from build123d import *

# Parameters (mm, degrees)
BOSS_EXTRU_1_DEPTH      = 13
BOSS_EXTRU_2_DEPTH      = 8
ESQUISSE4_R             = 5.5
BOSS_EXTRU_3_DEPTH      = 55
ENL_V_START             = -30
ESQUISSE5_R             = 5.5
ESQUISSE5_R_2           = 3
ENL_V_MAT_EXTRU_1_DEPTH = 30


with BuildPart() as part:
    # Esquisse1 → Boss.-Extru.1 (new body)
    with BuildSketch(Plane.XY):
        with BuildLine():
            Line((10.329521935, 9.6), (71.2270063, 5.135702408))
            ThreePointArc((71.2270063, 5.135702408), (76, 0), (71.2270063, -5.135702408))
            Line((71.2270063, -5.135702408), (10.329521935, -9.6))
            ThreePointArc((10.329521935, -9.6), (0, 0), (10.329521935, 9.6))
        make_face()
    extrude(amount=BOSS_EXTRU_1_DEPTH)

    # Esquisse3 → Boss.-Extru.2 (add)
    with BuildSketch(Plane.XY.offset(13)):
        with BuildLine():
            Line((71.263562407, 5.634364269), (10.366078041, 10.09866186))
            ThreePointArc((10.366078041, 10.09866186), (-0.5, 0), (10.366078041, -10.09866186))
            Line((10.366078041, -10.09866186), (71.263562407, -5.634364269))
            ThreePointArc((71.263562407, -5.634364269), (76.5, 0), (71.263562407, 5.634364269))
        make_face()
    extrude(amount=BOSS_EXTRU_2_DEPTH)

    # Esquisse4 → Boss.-Extru.3 (add)
    with BuildSketch(Plane.XY.offset(21)):
        with Locations((9.625761224, 0)):
            Circle(ESQUISSE4_R)
    extrude(amount=BOSS_EXTRU_3_DEPTH)

    # Esquisse5 → Enlèv. mat.-Extru.1 (cut)
    with BuildSketch(Plane.XY.offset(76).offset(ENL_V_START)):
        with Locations((9.625761224, 0)):
            Circle(ESQUISSE5_R)
        with Locations((9.625761224, 0)):
            Circle(ESQUISSE5_R_2, mode=Mode.SUBTRACT)
    extrude(amount=ENL_V_MAT_EXTRU_1_DEPTH, mode=Mode.SUBTRACT)


solid = part.part
Part model, mm, in its own coordinate system. A direction names the side the tool comes from. Coordinates: 2 decimals unless noted, no trailing zeros. Write each loop counter-clockwise with the first axis right and the second up, starting at its lowest first coordinate (ties: lowest second). Pieces come first, ordered by that corner, then holes. Notation, with made-up numbers: M -10,-15 L 3,-15 A19 cw 3,10 Z; hole C 61,-11 d5. An arc over 180 degrees is marked long. Return JSON: item names as keys, results as strings.
1. Saw through at B-B, the plane y = 0. Write the cut outline in (x, z), then the cut area to 3 significant figures.
Determined:
{"outline": "M -0.5,13 L 0,13 L 0,0 L 76,0 L 76,13 L 76.5,13 L 76.5,21 L 15.13,21 L 15.13,46 L 12.63,46 L 12.63,76 L 6.63,76 L 6.63,46 L 4.13,46 L 4.13,21 L -0.5,21 Z", "area": "2,060 mm²"}
2. 3-axis set-ups, long thin cutter, end or side, ignore diameter. For faces 1 (the face through (41.205, -7.337, 6.409)), 2 (the face through (6.63, 0.13, 60.79)), 3 (the face through (76.5, -0.1, 16.9)), 4 (the face through (40.35, 7.4, 6.41)), 5 (the face through (76, 0, 6)): which of +Z, -Z, +X, -X, +Y, -Y reach the whole face in a straight line?
Determined:
{"face 1": "-Z, +X, -Y", "face 2": "+Z", "face 3": "+Z, -Z, +X", "face 4": "-Z, +X, +Y", "face 5": "-Z, +X"}
3. Probe L1, parallel to Z at x = 73, y = -1.5; L2, parallel to Z at x = 70.5, y = 5.5; L3, parallel to Y at x = 61.5, z = 5.5. List the from-to ranges inside material, lowest first.
Determined:
{"L1": "0 to 21", "L2": "13 to 21", "L3": "-5.85 to 5.85"}
4. Flat gauge pins, fed straight in: pin 1 Ø10 at (x, y) = (49, 1.5) entering from -Z; pin 2 Ø4 at (x, z) = (16.5, 43) entering from -Y; pin 3 Ø1 at (y, z) = (-1.5, 56.5) entering from -X; pin 4 Ø5 at (x, z) = (9.5, 55) entering from -Y. Where does each tip first touch, or does it go through?
Determined:
{"pin 1": "z = 0", "pin 2": "y = -2.55", "pin 3": "x = 6.8", "pin 4": "y = -3"}
5. Saw through at A-A, the plane x = 35.5. Write the cut outline in (y, z).
Determined:
{"outline": "M -8.26,13 L -7.75,13 L -7.75,0 L 7.75,0 L 7.75,13 L 8.26,13 L 8.26,21 L -8.26,21 Z"}
6. Saw through at C-C, the plane z = 56.5. Write the cut outline in (x, y).
Determined:
{"outline": "C 9.63,0 d6"}
7. Saw through at D-D, the plane x = 18.5. Write the cut outline in (y, z), then the cut area to 3 significant figures.
Determined:
{"outline": "M -9.5,13 L -9,13 L -9,0 L 9,0 L 9,13 L 9.5,13 L 9.5,21 L -9.5,21 Z", "area": "386 mm²"}
